Work out the finished part from the listing and answer in its coordinate system (mm). A direction names the side the tool comes from. Coordinates: 2 decimals unless noted, no trailing zeros. Write each loop counter-clockwise with the first axis right and the second up, starting at its lowest first coordinate (ties: lowest second). Pieces come first, ordered by that corner, then holes. Notation, with made-up numbers: M 53.25,-10.75 L 75.25,-10.75 A38 ccw 75.25,27.25 Z; hole C 86.5,-34.75 d2. An arc over 180 degrees is marked long. Answer as CSV lines item,"result". Start each with the question number.
(1) For faces 1 (the flat face through (6.4, -4, 3.4)), 2 (the conical face through (0.174, 8.301, -0.02)), determine the directions among +Z, -Z, +X, -X, +Y, -Y from which every point of the face is accessible in a straight line to the end or side of a thin tool.
(2) A cutting plane is placed at A-A on x = 85.5. Give the vertices of the cut face in (y, z), then the cut area to 3 significant figures.
(3) Find the intervals of material crossed by L1, parallel to Y at x = 67.5, z = 3; L2, parallel to X at y = 2.5, z = 5; L3, parallel to Y at x = 36.5, z = 2.75, in increasing order. Write a range as [from, to].
(4) Flat-ended cylindrical pins translate along their axes: P1, Ø8, axis at y = -1.5, z = -6, coming from the +X side; P2, Ø4, axis at x = 37, z = -6, coming from the +Y side; P3, Ø3, axis at x = 38.5, z = -3.5, coming from the -Y side; P4, Ø8, axis at x = 13, y = 1, coming from the +Z side. Find the tip coordinate at first contact, or state that the pin passes through.
from build123d import *

# Parameters (mm, degrees)
BASEHEAD_DEPTH = 6.4


with BuildPart() as part:
    # Sketch1 → BaseHead (new body)
    with BuildSketch(Plane(origin=(0, 0, 0), x_dir=(0, 0, -1), z_dir=(1, 0, 0))):
        Polygon((8, 4.618802154), (8, -4.618802154), (0, -9.237604307), (-8, -4.618802154), (-8, 4.618802154), (0, 9.237604307), align=None)
    extrude(amount=BASEHEAD_DEPTH)

    # BodySke → BaseBody (revolve)
    with BuildSketch(Plane.XY, mode=Mode.PRIVATE) as basebody_sk:
        Polygon((0, 0), (106.4, 0), (106.4, 4.172), (105.572, 5), (0, 5), align=None)
    revolve(basebody_sk.sketch.rotate(Axis((0, 0, 0), (1, 0, 0)), 90), axis=Axis((0, 0, 0), (1, 0, 0)))

    # Sketch3 → HeadChamfer (revolve, cut)
    with BuildSketch(Plane.XY):
        Polygon((0, 8), (3.601282526, 14.237604307), (3.601282526, 19.237604307), (-10, 19.237604307), (-10, 8), align=None)
    revolve(axis=Axis((0, 0, 0), (1, 0, 0)), mode=Mode.SUBTRACT)


solid = part.part
Here are the results:
1,face 1,"+X"
1,face 2,"-X, +Y"
2,outline,"C 0,0 d10"
2,area,"78.5 mm^2"
3,L1,"y = [-4, 4]"
3,L2,"x = [0, 6.4]"
3,L3,"y = [-4.18, 4.18]"
4,P1,"stops at x = 106.4"
4,P2,"stops at y = 3"
4,P3,"stops at y = -4.58"
4,P4,"stops at z = 5"
